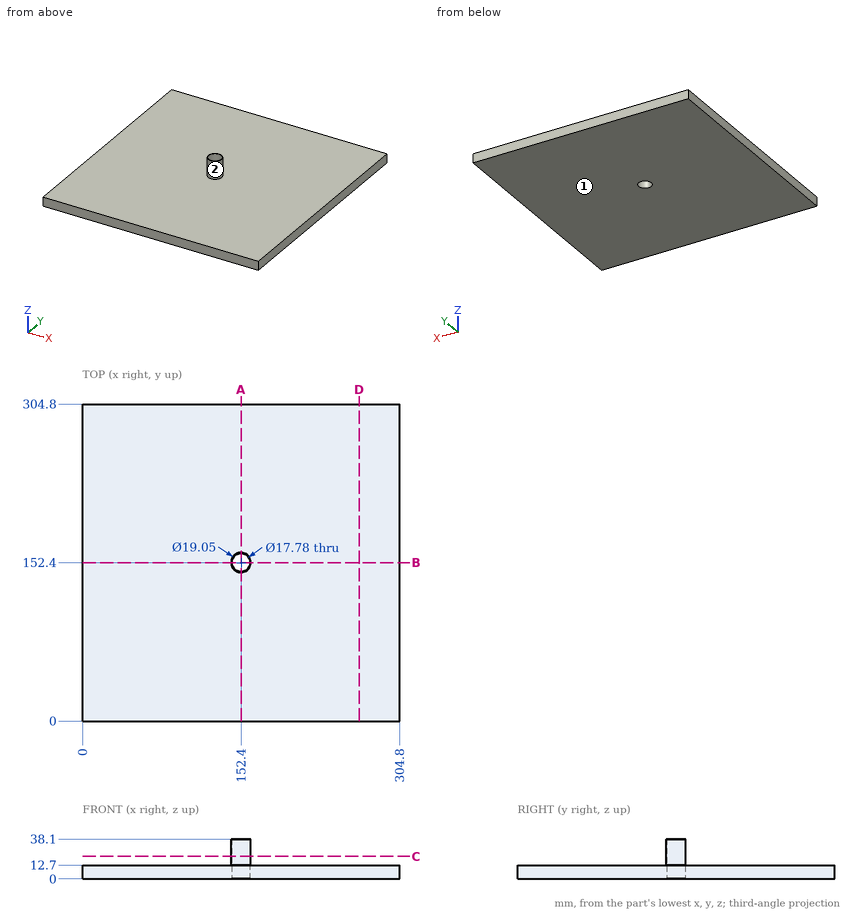
Design review of the part shown in the three views and the two pictorial views. Dimensions are in mm from the part's minimum x, y and z. A direction names the side the tool comes from. Round coordinates to 2 decimals unless told otherwise and drop trailing zeros. Loops run counter-clockwise (first coordinate to the right, second up) from the corner with the lowest first, then second, coordinate; pieces in that order, holes last. Notation, with made-up numbers: (7, 9) -> (30, 9) arc R20 ccw to (30, 27) -> close; hole circle Ø10 at (1.5, 9.25). An arc over 180 degrees is marked (long way). Return JSON: item names as keys, results as strings.
(1) Add section C-C on z = 21.5. Write out the cut boundary in (x, y) (3 decimals), plus the area to 3 significant figures.
Solved:
{"outline": "circle Ø19.05 at (152.4, 152.4); hole circle Ø17.78 at (152.4, 152.4)", "area": "36.7 mm2"}
(2) For the marked faces 1 and 2, list the 3-axis set-ups (+Z, -Z, +X, -X, +Y, -Y) from which the entire face can be reached by the end or side of a thin tool; tool diameter is ignored.
Solved:
{"face 1": "-Z, +X, -X, +Y, -Y", "face 2": "+Z"}
(3) For pin 1 (10.5 mm diameter, centred on x = 152.4, y = 152.4, fed in from -Z) (3 decimals); pin 2 (10 mm diameter, centred on x = 153, z = 16.5, fed in from +Y); pin 3 (4 mm diameter, centred on x = 202, y = 106, fed in from +Z), all flat-tipped, find the tip position at first contact; note any pin that passes through.
Solved:
{"pin 1": "through", "pin 2": "y = 304.8", "pin 3": "z = 12.7"}
(4) Add section A-A on x = 152.4. Write out the cut boundary in (y, z) (3 decimals).
Solved:
{"outline": "(0, 0) -> (143.51, 0) -> (143.51, 38.1) -> (142.875, 38.1) -> (142.875, 12.7) -> (0, 12.7) -> close; (161.29, 0) -> (304.8, 0) -> (304.8, 12.7) -> (161.925, 12.7) -> (161.925, 38.1) -> (161.29, 38.1) -> close"}
(5) Add section D-D on x = 266. Write out the cut boundary in (y, z).
Solved:
{"outline": "(0, 0) -> (304.8, 0) -> (304.8, 12.7) -> (0, 12.7) -> close"}
(6) For line 1 (Y direction, x = 152.4, z = 30) (3 decimals); line 2 (X direction, y = 152, z = 10); line 3 (Z direction, x = 79.5, y = 228), list the stretches that pass through material, from the lowest coordinate up.
Solved:
{"line 1": "142.875 to 143.51, 161.29 to 161.925", "line 2": "0 to 143.52, 161.28 to 304.8", "line 3": "0 to 12.7"}
